```python
from build123d import *

# Parameters (mm, degrees)
BOSS_EXTRUDE1_DEPTH = 60
SKETCH2_W           = 1.5
SKETCH2_H           = 3.5
BOSS_EXTRUDE2_DEPTH = 0.7
SKETCH2_2_W         = 1.5
SKETCH2_2_H         = 3.5
BOSS_EXTRUDE3_DEPTH = 0.25
CHAMFER1_SIZE       = 0.6
CHAMFER2_SIZE       = 0.6
BOSS_EXTRUDE4_DEPTH = 10
CHAMFER3_SIZE       = 1
CHAMFER4_SIZE       = 0.25


with BuildPart() as part:
    # Sketch1 → Boss-Extrude1 (new body)
    with BuildSketch(Plane(origin=(0, 0, 0), x_dir=(1, 0, 0), z_dir=(0, 1, 0))):
        with BuildLine():
            Line((-3.112876483, -2), (3.112876483, -2))
            ThreePointArc((3.112876483, -2), (0, 3.7), (-3.112876483, -2))
        make_face()
    extrude(amount=BOSS_EXTRUDE1_DEPTH)



with BuildPart() as body_2:
    # Sketch2 → Boss-Extrude2 (new body)
    with BuildSketch(Plane(origin=(0, 0, -3.7), x_dir=(-1, 0, 0), z_dir=(0, 0, -1))):
        with Locations((0, 47.75)):
            Rectangle(SKETCH2_W, SKETCH2_H)
    extrude(amount=BOSS_EXTRUDE2_DEPTH)


with BuildPart() as part_1:
    add(part.part)

    add(body_2.part)  # Boss-Extrude3 merges body 2
    # Sketch2<2> → Boss-Extrude3 (add)
    with BuildSketch(Plane(origin=(0, 0, -3.7), x_dir=(-1, 0, 0), z_dir=(0, 0, -1))):
        with Locations((0, 47.75)):
            Rectangle(SKETCH2_2_W, SKETCH2_2_H)
    extrude(amount=-BOSS_EXTRUDE3_DEPTH)

    # Chamfer1
    chamfer1_edges = [part_1.edges().sort_by_distance(p)[0] for p in [
        (0, 49.5, -4.4),
    ]]
    chamfer(chamfer1_edges, length=CHAMFER1_SIZE)

    # Chamfer2
    chamfer2_edges = [part_1.edges().sort_by_distance(p)[0] for p in [
        (0, 46, -4.4),
    ]]
    chamfer(chamfer2_edges, length=CHAMFER2_SIZE)

    # Sketch3 → Boss-Extrude4 (add)
    with BuildSketch(Plane(origin=(0, 60, 0), x_dir=(1, 0, 0), z_dir=(0, 1, 0))):
        with BuildLine():
            Line((-2.569533032, -3), (2.569533032, -3))
            ThreePointArc((2.569533032, -3), (0, 3.95), (-2.569533032, -3))
        make_face()
    extrude(amount=BOSS_EXTRUDE4_DEPTH)

    # Chamfer3
    chamfer3_edges = [part_1.edges().sort_by_distance(p)[0] for p in [
        (0, 60, 3),
    ]]
    chamfer(chamfer3_edges, length=CHAMFER3_SIZE - 0.0001)  # a hair under: the kernel refuses the full size

    # Chamfer4
    chamfer4_edges = [part_1.edges().sort_by_distance(p)[0] for p in [
        (0, 60, -3.95),
    ]]
    chamfer(chamfer4_edges, length=CHAMFER4_SIZE - 0.0001)  # a hair under: the kernel refuses the full size


solid = part_1.part
```
Input: part model. Units: mm. Frame: model coordinates. A direction names the side the tool comes from. Coordinates: 2 decimals unless noted, no trailing zeros. Loops run counter-clockwise (first coordinate to the right, second up) from the corner with the lowest first, then second, coordinate; pieces in that order, holes last. Notation, with made-up numbers: (15, 14.25) - (21, 14.25) arc R11 cw to (21, 22.25) - close; hole circle Ø2 at (70, -13). An arc over 180 degrees is marked (long way). Answer in a Markdown table with one row per item.
(1) Set-up query: faces 1 (the face through (0, 30, 2)), 2 (the face through (0, 70, -1)). Return all of +Z, -Z, +X, -X, +Y, -Y with unobstructed straight access to the full face (end or side cutting, diameter ignored); none if empty.
Model answer:
| item | result |
|---|---|
| face 1 | +Z, +X, -X, -Y |
| face 2 | +Z, -Z, +X, -X, +Y |
(2) Pin query (flat end, axial travel): P1, Ø3, axis at x = -0.5, y = 12, coming from the -Z side; P2, Ø4, axis at y = 26, z = 1, coming from the +X side; P3, Ø0.6, axis at y = 48.5, z = -4, coming from the -X side. Return the tip coordinate at first contact, or that it passes through.
Model answer:
| item | result |
|---|---|
| P1 | stops at z = -3.7 |
| P2 | stops at x = 3.7 |
| P3 | stops at x = -0.75 |
(3) Cut plane C-C on y = 25. Output: boundary loops of the cut face in (x, z).
Model answer:
| item | result |
|---|---|
| outline | (-3.11, 2) arc R3.7 ccw (long way) to (3.11, 2) - close |
(4) Material intervals for L1, parallel to Z at x = 2, y = 31; L2, parallel to X at y = 67, z = -3; L3, parallel to Z at x = 0, y = 36, sorted ascending. Write a range as from..to.
Model answer:
| item | result |
|---|---|
| L1 | z = -3.11..2 |
| L2 | x = -2.57..2.57 |
| L3 | z = -3.7..2 |
